For this review, take the finished solid that the model builds, in its own axes (mm). A direction names the side the tool comes from. Coordinates: 2 decimals unless noted, no trailing zeros. Write each loop counter-clockwise with the first axis right and the second up, starting at its lowest first coordinate (ties: lowest second). Pieces come first, ordered by that corner, then holes.
1) We need section B-B on z = 4.25. Give the number of separate pieces and of enclosed holes in the cut face, then the cut area to 3 significant figures.
2) Mouldability with a two-part tool opening along X and no side actions: class faces 3 (the face through (-44, -38.786, 5)), 4 (the face through (-44, 43.764, 5)), 5 (the face through (-2, 1, 0)), 6 (the face through (-169.284, 48.89, 4.829)) as pulls with the +X half, pulls with the -X half, needs draft (parallel to the pull), parting line crosses it, or undercut.
3) To check wall thickness, follow line 1 along Y through (x, z) = (49, 6.75); line 2 along Y through (x, z) = (-151, 3.5); line 3 along X through (y, z) = (-43, 7.5). State the ranges of each line that lie inside material, in increasing order.
4) Insertion check: P1, Ø10, axis at x = -115.5, y = -33, coming from the -Z side. The pin has a flat end and moves straight along its axis. Give the tip position at first contact, or say it passes through.
5) We need section A-A on x = 132.5. Write out the cut boundary in (y, z) (3 decimals).
6) For faces 1 (the face through (-2, 50.8, 5)), 2 (the face through (127, 43.764, 5)), list the 3-axis set-ups (+Z, -Z, +X, -X, +Y, -Y) from which the entire face can be reached by the end or side of a thin tool; tool diameter is ignored.
from build123d import *

# Parameters (mm, degrees)
SKETCH1_W                  = 342.1888
SKETCH1_H                  = 101.6
BOSS_EXTRUDE1_DEPTH        = 9.525
F_10_CLEARANCE_SLOT1_DEPTH = 9.525
FILLET1_R                  = 6.35


# Read off the part's stored shape, not the designer's step: #10 Clearance Slot1
with BuildPart() as part:
    # Sketch1 → Boss-Extrude1 (new body)
    with BuildSketch(Plane.XY):
        Rectangle(SKETCH1_W, SKETCH1_H)
    extrude(amount=BOSS_EXTRUDE1_DEPTH)

    # #10 Clearance Slot1 outline → #10 Clearance Slot1 (cut)
    with BuildSketch(Plane.XY):
        with BuildLine():
            Line((-149.0472, 38.7858), (-104.5972, 38.7858))
            ThreePointArc((-104.5972, 38.7858), (-102.108, 41.275), (-104.5972, 43.7642))
            Line((-104.5972, 43.7642), (-149.0472, 43.7642))
            ThreePointArc((-149.0472, 43.7642), (-151.5364, 41.275), (-149.0472, 38.7858))
        make_face()
        with BuildLine():
            ThreePointArc((-22.0472, 38.7858), (-19.558, 41.275), (-22.0472, 43.7642))
            Line((-22.0472, 43.7642), (-66.4972, 43.7642))
            ThreePointArc((-66.4972, 43.7642), (-68.9864, 41.275), (-66.4972, 38.7858))
            Line((-66.4972, 38.7858), (-22.0472, 38.7858))
        make_face()
        with BuildLine():
            ThreePointArc((66.4972, 38.7858), (68.9864, 41.275), (66.4972, 43.7642))
            Line((66.4972, 43.7642), (22.0472, 43.7642))
            ThreePointArc((22.0472, 43.7642), (19.558, 41.275), (22.0472, 38.7858))
            Line((22.0472, 38.7858), (66.4972, 38.7858))
        make_face()
        with BuildLine():
            ThreePointArc((149.0472, 38.7858), (151.5364, 41.275), (149.0472, 43.7642))
            Line((149.0472, 43.7642), (104.5972, 43.7642))
            ThreePointArc((104.5972, 43.7642), (102.108, 41.275), (104.5972, 38.7858))
            Line((104.5972, 38.7858), (149.0472, 38.7858))
        make_face()
        with BuildLine():
            Line((104.5972, -43.7642), (149.0472, -43.7642))
            ThreePointArc((149.0472, -43.7642), (151.5364, -41.275), (149.0472, -38.7858))
            Line((149.0472, -38.7858), (104.5972, -38.7858))
            ThreePointArc((104.5972, -38.7858), (102.108, -41.275), (104.5972, -43.7642))
        make_face()
        with BuildLine():
            ThreePointArc((66.4972, -43.7642), (68.9864, -41.275), (66.4972, -38.7858))
            Line((66.4972, -38.7858), (22.0472, -38.7858))
            ThreePointArc((22.0472, -38.7858), (19.558, -41.275), (22.0472, -43.7642))
            Line((22.0472, -43.7642), (66.4972, -43.7642))
        make_face()
        with BuildLine():
            ThreePointArc((-22.0472, -43.7642), (-19.558, -41.275), (-22.0472, -38.7858))
            Line((-22.0472, -38.7858), (-66.4972, -38.7858))
            ThreePointArc((-66.4972, -38.7858), (-68.9864, -41.275), (-66.4972, -43.7642))
            Line((-66.4972, -43.7642), (-22.0472, -43.7642))
        make_face()
        with BuildLine():
            ThreePointArc((-104.5972, -43.7642), (-102.108, -41.275), (-104.5972, -38.7858))
            Line((-104.5972, -38.7858), (-149.0472, -38.7858))
            ThreePointArc((-149.0472, -38.7858), (-151.5364, -41.275), (-149.0472, -43.7642))
            Line((-149.0472, -43.7642), (-104.5972, -43.7642))
        make_face()
    extrude(amount=F_10_CLEARANCE_SLOT1_DEPTH, mode=Mode.SUBTRACT)

    # Fillet1
    fillet1_edges = [part.edges().sort_by_distance(p)[0] for p in [
        (-171.0944, 50.8, 4.7625),
        (171.0944, 50.8, 4.7625),
        (171.0944, -50.8, 4.7625),
        (-171.0944, -50.8, 4.7625),
    ]]
    fillet(fillet1_edges, radius=FILLET1_R)


solid = part.part
Result:
1. separate pieces: 1
1. enclosed holes: 8
1. area: 32,800 mm2
2. face 3: undercut
2. face 4: undercut
2. face 5: needs draft
2. face 6: pulls with the -X half
3. line 1: y = -50.8 to -43.76, -38.79 to 38.79, 43.76 to 50.8
3. line 2: y = -50.8 to -42.82, -39.73 to 39.73, 42.82 to 50.8
3. line 3: x = -171.09 to -150.84, -102.8 to -68.29, -20.25 to 20.25, 68.29 to 102.8, 150.84 to 171.09
4. P1: stops at z = 0
5. outline: (-50.8, 0) - (-43.764, 0) - (-43.764, 9.525) - (-50.8, 9.525) - close; (-38.786, 0) - (38.786, 0) - (38.786, 9.525) - (-38.786, 9.525) - close; (43.764, 0) - (50.8, 0) - (50.8, 9.525) - (43.764, 9.525) - close
6. face 1: +Z, -Z, +X, -X, +Y
6. face 2: +Z, -Z
